Autodesk Inventor part; units mm, degrees
ref_plane "YZ Plane" through (0, 0, 0) normal (1, 0, 0) x (0, 1, 0)
ref_plane "XZ Plane" through (0, 0, 0) normal (0, 1, 0) x (-1, 0, 0)
ref_plane "XY Plane" through (0, 0, 0) normal (0, 0, 1) x (1, 0, 0)
sketch "Boceto1" plane through (0, 0, 0) normal (0, 0, 1) x (1, 0, 0)
  circle A0 centre (0, 0) radius 6.5
  dimension "d0" = 13
extrude "Extrusión1" add sketch "Boceto1" along normal blind 8.25
sketch "Boceto2" plane through (0, 0, 8.25) normal (0, 0, 1) x (1, 0, 0)
  circle A0 centre (0, 0) radius 6.5
  circle A1 centre (0, 0) radius 7.35
  dimension "d3" = 14.7
extrude "Extrusión2" add sketch "Boceto2" along normal blind 29.75 contours A0 | A1
sketch "Boceto3" plane through (0, 0, 38) normal (0, 0, 1) x (1, 0, 0)
  circle A0 centre (0, 0) radius 7.35
  circle A1 centre (0, 0) radius 5.65
  dimension "d6" = 11.3
extrude "Extrusión3" add sketch "Boceto3" along normal blind 4.7 contours A1
sketch "Boceto4" plane through (0, 0, 0) normal (1, 0, 0) x (0, 1, 0)
  line L0 (5.65, 42.7) -> (-5.65, 42.7)
  line L1 (7.35, 38) -> (-7.35, 38)
  line L2 (5.65, 42.7) -> (7.35, 38)
  line L3 (5.65, 38) -> (5.65, 42.7)
  line L4 (0, 42.7) -> (0, 50.6655) construction
  point P0 (0, 0)
revolve "Revolución1" add sketch "Boceto4" angle 360 about axis through (0, 0, 42.7) along (0, 0, 1)
sketch "Boceto7" plane through (0, 0, 0) normal (1, 0, 0) x (0, 1, 0)
  line L0 (5.65, 42.7) -> (-5.65, 42.7)
  line L1 (0, 42.7) -> (4.95, 42.7) construction
  line L2 (0, 42.7) -> (0, 62.2)
  line L3 (0, 62.2) -> (3.9, 62.2)
  line L4 (3.9, 62.2) -> (4.95, 42.7)
  point P0 (0, 0)
  dimension "d13" = 4.95
  dimension "d14" = 19.5
  dimension "d15" = 3.9
revolve "Revolución2" add sketch "Boceto7" angle 360 about axis through (0, 0, 42.7) along (0, 0, 1)
sketch "Boceto8" plane through (0, 0, 62.2) normal (0, 0, 1) x (1, 0, 0)
  circle A0 centre (0, 0) radius 3.9
  circle A1 centre (0, 0) radius 2.15
  dimension "d17" = 4.3
extrude "Extrusión5" add sketch "Boceto8" along normal blind 82 contours A1
sketch "Boceto9" plane through (0, 0, 144.2) normal (0, 0, 1) x (1, 0, 0)
  circle A0 centre (0, 0) radius 2.15
  circle A1 centre (0, 0) radius 1.95
  dimension "d20" = 3.9
extrude "Extrusión6" add sketch "Boceto9" along normal blind 238 contours A1
sketch "Boceto10" plane through (0, 0, 382.2) normal (0, 0, 1) x (1, 0, 0)
  circle A0 centre (0, 0) radius 1.95
  circle A1 centre (0, 0) radius 2.9
  dimension "d23" = 5.8
extrude "Extrusión7" add sketch "Boceto10" along normal blind 13.4 contours A0 | A1
fillet "Empalme1" radius 2 1 edges at (-2.9, 0, 395.6)
fillet "Empalme2" radius 0.5 1 edges at (-2.9, 0, 382.2)
sketch "Boceto11" plane through (0, 0, 0) normal (0, 0, -1) x (-1, 0, 0)
  circle A0 centre (0, 0) radius 6.5
  circle A1 centre (0, 0) radius 3.05
  dimension "d28" = 6.1
hole "Hole1" at (0, 0, 0) direction (0, 0, 1) diameter 6.401 depth 15
sketch "Boceto12" plane through (0, 0, 15) normal (0, 0, -1) x (-1, 0, 0)
  circle A0 centre (0, 0) radius 3.2005
  circle A1 centre (0, 0) radius 0.25
  dimension "d36" = 0.5
extrude "Extrusión8" cut sketch "Boceto12" against normal blind 10 contours A1
properties part number "nagoya771"
Input: part model. Units: mm. Frame: model coordinates. A direction names the side the tool comes from. Give positions to 0.01 mm unless a question says otherwise; leave off trailing zeros. Loops run counter-clockwise (first coordinate to the right, second up) from the corner with the lowest first, then second, coordinate; pieces in that order, holes last. Notation, with made-up numbers: (25.25, 4) -> (82.25, 4) arc R26 ccw to (82.25, 38) -> close; hole circle Ø8 at (88, 23.5). An arc over 180 degrees is marked (long way). Use a Markdown table: item, result.
Q1. First-contact query: P1, Ø6, axis at y = -2, z = 96, coming from the -X side; P2, Ø3, axis at x = 0.5, y = -0.5, coming from the -Z side; P3, Ø4, axis at x = 0, z = 224, coming from the -Y side. Flat tips, straight axial feed; report the tip coordinate or a pass-through.
Entries:
| item | result |
|---|---|
| P1 | stops at x = -2.15 |
| P2 | stops at z = 15 |
| P3 | stops at y = -1.95 |
Q2. Access query for faces 1 (the flat face through (1, 0, 15)), 2 (the conical face through (1.7, 5.5, 42.4)). Directions: +Z, -Z, +X, -X, +Y, -Y. A direction counts if a zero-diameter tool reaches every point of the face in a straight line with its end or side. Return the directions, or none.
Entries:
| item | result |
|---|---|
| face 1 | -Z |
| face 2 | +Z |
Q3. Section query A-A, the plane z = 252.5. Return the cut outline in (x, y).
Entries:
| item | result |
|---|---|
| outline | circle Ø3.9 at (0, 0) |
Q4. Pull-direction query (Z, two-part tool) for faces 3 (the cylindrical face through (-1.593, 7.175, 22.917)), 4 (the flat face through (2, 2, 62.2)), 5 (the flat face through (3, -6, 8.25)), 6 (the flat face through (2, -5, 42.7)); classes: pulls with the +Z half, pulls with the -Z half, needs draft (parallel to the pull), parting line crosses it, or undercut.
Entries:
| item | result |
|---|---|
| face 3 | needs draft |
| face 4 | undercut |
| face 5 | pulls with the -Z half |
| face 6 | pulls with the +Z half |
Q5. Ray query, probe 1 along Y at (x, z) = (0, 23.25); probe 2 along Y at (x, z) = (0, 8); probe 3 along Z at (x, y) = (0.25, -0.5). Return the intervals inside material, ascending. Write a range as from..to.
Entries:
| item | result |
|---|---|
| probe 1 | y = -7.35..-0.25, 0.25..7.35 |
| probe 2 | y = -6.5..-3.2, 3.2..6.5 |
| probe 3 | z = 15..395.6 |
